The listing builds one solid part. Answer for the finished solid, in the listing's coordinates (mm). A direction names the side the tool comes from. Give positions to 0.01 mm unless a question says otherwise; leave off trailing zeros. Write each loop counter-clockwise with the first axis right and the second up, starting at its lowest first coordinate (ties: lowest second). Pieces come first, ordered by that corner, then holes. Notation, with made-up numbers: (24, 53.5) -> (28, 53.5) arc R17 cw to (28, 77.5) -> close; hole circle Ø2 at (-35, 58.25). An arc over 180 degrees is marked (long way). One line per question, with ' | ' between items.
from build123d import *

# Parameters (mm, degrees)
BOSS_EXTRUDE1_DEPTH = 55
SKETCH2_R           = 2
CUT_EXTRUDE1_DEPTH  = 72.763500472
CUT_EXTRUDE2_DEPTH  = 3
SKETCH4_R           = 4.2
CUT_EXTRUDE3_DEPTH  = 72.763500472
SKETCH5_R           = 9
CUT_EXTRUDE4_DEPTH  = 3
SKETCH6_R           = 4.2
CUT_EXTRUDE5_DEPTH  = 10
SKETCH7_W           = 16.5
SKETCH7_H           = 30
CUT_EXTRUDE6_DEPTH  = 7
BOSS_EXTRUDE2_START = 10
SKETCH8_W           = 55
SKETCH8_H           = 40
SKETCH8_R           = 4.2
BOSS_EXTRUDE2_DEPTH = 10
CHAMFER1_SIZE       = 2


with BuildPart() as part:
    # Sketch1 → Boss-Extrude1 (new body)
    with BuildSketch(Plane.XY):
        Polygon((0, 0), (35, 0), (35, 40), (25, 40), (25, 10), (0, 10), (-25, 10), (-25, 40), (-35, 40), (-35, 0), align=None)
    extrude(amount=BOSS_EXTRUDE1_DEPTH)

    # Sketch2 → Cut-Extrude1 (cut, through all)
    with BuildSketch(Plane(origin=(0, 10, 0), x_dir=(1, 0, 0), z_dir=(0, 1, 0))):
        with Locations(Location((-15, -12.5, 0), (0, 0, 180))):
            Circle(SKETCH2_R)
        with Locations(Location((-15, -22.5, 0), (0, 0, 180))):
            Circle(SKETCH2_R)
        with Locations(Location((15, -12.5, 0), (0, 0, 180))):
            Circle(SKETCH2_R)
        with Locations(Location((15, -22.5, 0), (0, 0, 180))):
            Circle(SKETCH2_R)
        with Locations(Location((15, -32.5, 0), (0, 0, 180))):
            Circle(SKETCH2_R)
        with Locations(Location((-15, -32.5, 0), (0, 0, 180))):
            Circle(SKETCH2_R)
        with Locations(Location((-15, -42.5, 0), (0, 0, 180))):
            Circle(SKETCH2_R)
        with Locations(Location((15, -42.5, 0), (0, 0, 180))):
            Circle(SKETCH2_R)
    extrude(amount=-CUT_EXTRUDE1_DEPTH, mode=Mode.SUBTRACT)

    # Sketch3 → Cut-Extrude2 (cut)
    with BuildSketch(Plane.XZ):
        Polygon((-10.958548116, 12.5), (-12.979274058, 16), (-17.020725942, 16), (-19.041451884, 12.5), (-17.020725942, 9), (-12.979274058, 9), align=None)
        Polygon((-10.958548116, 22.5), (-12.979274058, 26), (-17.020725942, 26), (-19.041451884, 22.5), (-17.020725942, 19), (-12.979274058, 19), align=None)
        Polygon((-10.958548116, 32.5), (-12.979274058, 36), (-17.020725942, 36), (-19.041451884, 32.5), (-17.020725942, 29), (-12.979274058, 29), align=None)
        Polygon((-10.958548116, 42.5), (-12.979274058, 46), (-17.020725942, 46), (-19.041451884, 42.5), (-17.020725942, 39), (-12.979274058, 39), align=None)
        Polygon((19.041451884, 42.5), (17.020725942, 46), (12.979274058, 46), (10.958548116, 42.5), (12.979274058, 39), (17.020725942, 39), align=None)
        Polygon((19.041451884, 32.5), (17.020725942, 36), (12.979274058, 36), (10.958548116, 32.5), (12.979274058, 29), (17.020725942, 29), align=None)
        Polygon((19.041451884, 22.5), (17.020725942, 26), (12.979274058, 26), (10.958548116, 22.5), (12.979274058, 19), (17.020725942, 19), align=None)
        Polygon((19.041451884, 12.5), (17.020725942, 16), (12.979274058, 16), (10.958548116, 12.5), (12.979274058, 9), (17.020725942, 9), align=None)
    extrude(amount=-CUT_EXTRUDE2_DEPTH, mode=Mode.SUBTRACT)

    # Sketch4 → Cut-Extrude3 (cut, through all)
    with BuildSketch(Plane(origin=(0, 10, 0), x_dir=(1, 0, 0), z_dir=(0, 1, 0))):
        with Locations(Location((0, -27.5, 0), (0, 0, 180))):
            Circle(SKETCH4_R)
    extrude(amount=-CUT_EXTRUDE3_DEPTH, mode=Mode.SUBTRACT)

    # Sketch5 → Cut-Extrude4 (cut)
    with BuildSketch(Plane(origin=(0, 10, 0), x_dir=(1, 0, 0), z_dir=(0, 1, 0))):
        with Locations(Location((0, -27.5, 0), (0, 0, 180))):
            Circle(SKETCH5_R)
    extrude(amount=-CUT_EXTRUDE4_DEPTH, mode=Mode.SUBTRACT)

    # Sketch6 → Cut-Extrude5 (cut)
    with BuildSketch(Plane(origin=(35, 0, 0), x_dir=(0, 0, -1), z_dir=(1, 0, 0))):
        with Locations((-27.5, 20)):
            Circle(SKETCH6_R)
    extrude(amount=-CUT_EXTRUDE5_DEPTH, mode=Mode.SUBTRACT)

    # Sketch7 → Cut-Extrude6 (cut)
    with BuildSketch(Plane.ZY.offset(-25)):
        with Locations((27.5, 25)):
            Rectangle(SKETCH7_W, SKETCH7_H)
    extrude(amount=-CUT_EXTRUDE6_DEPTH, mode=Mode.SUBTRACT)

    # Sketch8 → Boss-Extrude2 (add)
    with BuildSketch(Plane(origin=(35, 0, 0), x_dir=(0, 0, -1), z_dir=(1, 0, 0)).offset(BOSS_EXTRUDE2_START)):
        with Locations((-27.5, 20)):
            Rectangle(SKETCH8_W, SKETCH8_H)
        with Locations((-27.5, 20)):
            Circle(SKETCH8_R, mode=Mode.SUBTRACT)
    extrude(amount=-BOSS_EXTRUDE2_DEPTH)

    # Chamfer1
    chamfer1_edges = [part.edges().sort_by_distance(p)[0] for p in [
        (-35, 20, 0),
        (-30, 40, 0),
        (35, 40, 0),
        (-35, 40, 27.5),
        (45, 20, 0),
        (45, 40, 27.5),
        (45, 20, 55),
        (-30, 40, 55),
        (-35, 20, 55),
        (35, 40, 55),
    ]]
    chamfer(chamfer1_edges, length=CHAMFER1_SIZE)


solid = part.part
Item 1: A tool of negligible diameter and unlimited length cuts with its end or side. For faces 4 (the face through (28, 25, 19.25)), 5 (the face through (15, 1, 36)), 6 (the face through (45, 15, 28)), from which of +Z, -Z, +X, -X, +Y, -Y can it reach the whole face along a straight path? Write none if from no direction.
Answers below:
face 4: +Y | face 5: -Y | face 6: +Z, -Z, +X, +Y, -Y
Item 2: Find section B-B (y = 20). Write down the section's boundary in (x, z).
Answers below:
outline: (-35, 2) -> (-33, 0) -> (-25, 0) -> (-25, 55) -> (-33, 55) -> (-35, 53) -> close; (25, 0) -> (43, 0) -> (45, 2) -> (45, 23.3) -> (32, 23.3) -> (32, 19.25) -> (25, 19.25) -> close; (25, 35.75) -> (32, 35.75) -> (32, 31.7) -> (45, 31.7) -> (45, 53) -> (43, 55) -> (25, 55) -> close
Item 3: Find section A-A (x = 0). Write down the section's boundary in (y, z).
Answers below:
outline: (0, 0) -> (10, 0) -> (10, 18.5) -> (7, 18.5) -> (7, 23.3) -> (0, 23.3) -> close; (0, 31.7) -> (7, 31.7) -> (7, 36.5) -> (10, 36.5) -> (10, 55) -> (0, 55) -> close
Item 4: Find section D-D (x = 35.5). Write down the section's boundary in (y, z).
Answers below:
outline: (0, 0) -> (38, 0) -> (40, 2) -> (40, 53) -> (38, 55) -> (0, 55) -> close; hole circle Ø8.4 at (20, 27.5)
Item 5: Flat-ended cylindrical pins translate along their axes: pin 1 (6.5 mm diameter, centred on x = 15, z = 22.5, fed in from +Y); pin 2 (3.5 mm diameter, centred on x = -15.5, z = 31.5, fed in from -Y). Find the tip coordinate at first contact, or state that the pin passes through.
Answers below:
pin 1: y = 10 | pin 2: y = 3
Item 6: Consider line 1 (Z direction, x = 15, y = 5); line 2 (Z direction, x = 0, y = 5.5); line 3 (X direction, y = 34.5, z = 33). Determine where each line is inside the solid, lowest interval first. Write a range as [from, to].
Answers below:
line 1: [0, 10.5], [14.5, 20.5], [24.5, 30.5], [34.5, 40.5], [44.5, 55] | line 2: [0, 23.3], [31.7, 55] | line 3: [-35, -25], [32, 45]
Item 7: Determine the mould class of faces 1 (the face through (38.591, 24.164, 28.047)), 2 (the face through (-12, 1.5, 10.7)), 3 (the face through (-33.6, 38.6, 53.8)) for opening direction Y: pulls with the +Y half, pulls with the -Y half, needs draft (parallel to the pull), parting line crosses it, or undercut.
Answers below:
face 1: undercut | face 2: needs draft | face 3: pulls with the +Y half
Item 8: Find section C-C (y = 32). Write down the section's boundary in (x, z), then the cut area to 3 significant figures.
Answers below:
outline: (-35, 2) -> (-33, 0) -> (-25, 0) -> (-25, 55) -> (-33, 55) -> (-35, 53) -> close; (25, 0) -> (43, 0) -> (45, 2) -> (45, 53) -> (43, 55) -> (25, 55) -> (25, 35.75) -> (32, 35.75) -> (32, 19.25) -> (25, 19.25) -> close | area: 1,530 mm²
